Autodesk Fusion 360 part; units mm, degrees
box "BoxPrimitive1" add length 20 width 33 height 3 placed x (0, 0, 1) y (1, 0, 0) z (0, 1, 0) at (0, 0, 0)
sketch "Sketch2" plane through (0, 0, 0) normal (0, -1, 0) x (1, 0, 0)
  line L0 (33, 20) -> (0, 20)
  line L1 (0, 20) -> (0, 0)
  line L2 (0, 0) -> (33, 0)
  line L3 (33, 0) -> (33, 20)
  line L4 (16.5, 20) -> (16.5, 0)
  line L5 (16.5, 0) -> (16.5, 1)
  line L6 (16.5, 1) -> (27, 1)
  line L7 (27, 1) -> (6, 1)
  line L8 (6, 1) -> (6, 13)
  line L9 (6, 13) -> (27, 13)
  line L10 (27, 13) -> (27, 1)
  dimension "d6" = 1
  dimension "d7" = 10.5
  dimension "d8" = 21
  dimension "d9" = 12
extrude "Extrude1" add sketch "Sketch2" along normal blind 3 contours L4 L6 L7 L9 L10 | L4 L7 L8 L9
sketch "Sketch3" plane through (0, -3, 0) normal (0, -1, 0) x (1, 0, 0)
  line L0 (27, 13) -> (6, 13)
  line L1 (6, 13) -> (6, 1)
  line L2 (6, 1) -> (27, 1)
  line L3 (27, 1) -> (27, 13)
  line L4 (16.5, 13) -> (16.5, 1)
  line L5 (6, 7) -> (27, 7)
cylinder "CylinderPrimitive1" add diameter 9 height 2 placed x (1, 0, 0) y (0, 0, 1) z (0, -1, 0) at (16.5, -3, 7)
cylinder "CylinderPrimitive2" cut diameter 1.37 height -2 placed x (1, 0, 0) y (0, 0, 1) z (0, -1, 0) at (16.5, -5, 7)
Can you work these out from the model? Positions are in its coordinate system, mm. A direction names the side the tool comes from. Give positions to 0.01 mm unless a question says otherwise; leave off trailing zeros. Loops run counter-clockwise (first coordinate to the right, second up) from the corner with the lowest first, then second, coordinate; pieces in that order, holes last. Notation, with made-up numbers: M 82,-30 L 93,-30 A24 cw 93,9 Z; hole C -38,-3.75 d10. An arc over 180 degrees is marked long. One line per question, with ' | ' between items. Start each with the question number.
Q1. If we mould it in two halves opening along X, with no side actions, what happens to faces 1 (the flat face through (0, 1, 10)), 2 (the flat face through (16, -3, 7)), 3 (the flat face through (16, 1, 20)), 4 (the flat face through (27, -1, 7))? For each: +X half, -X half, draft (parallel to the pull), parting line (faces both ways), or undercut.
Q2. For pin 1 Ø1.1 at (x, z) = (16.5, 7) entering from -Y; pin 2 Ø0.9 at (x, y) = (17, -2) entering from -Z; pin 3 Ø1.5 at (x, y) = (21, -1.5) entering from +Z, each with a flat end and sliding along its axis, tell me the tip position at first contact or that it passes through.
Q3. For faces 5 (the cylindrical face through (17.15, -4.01, 7.21)), 6 (the flat face through (6, -1, 7)), 7 (the flat face through (16, -1, 13)), which set-ups out of +Z, -Z, +X, -X, +Y, -Y let a thin tool reach every point of the face, with its end or its side?
Q4. If we section it at A-A (x = 16.5): Please give me the cut outline in (y, z) (3 decimals), plus the area to 3 significant figures.
Q5. If I drill on line 1 (Z direction, x = 16.5, y = -4.4) (3 decimals); line 2 (Y direction, x = 4.5, z = 16.75); line 3 (Y direction, x = 26.5, z = 1.5), over which ranges is the centre line in solid material (lowest first)? Write a range as from..to.
Q6. If we section it at B-B (z = 7): Please give me the cut outline in (x, y) (3 decimals), plus the area to 3 significant figures.
Q7. If we section it at D-D (z = 10.25): Please give me the cut outline in (x, y), plus the area to 3 significant figures.
Q8. If we section it at C-C (y = -4): Please give me the cut outline in (x, z) (3 decimals), plus the area to 3 significant figures.
Computed:
1) face 1: -X half | face 2: undercut | face 3: draft | face 4: +X half
2) pin 1: stops at y = -3 | pin 2: stops at z = 1 | pin 3: stops at z = 13
3) face 5: -Y | face 6: +Z, -Z, -X, -Y | face 7: +Z, +X, -X, -Y
4) outline: M -5,2.5 L -3,2.5 L -3,1 L 0,1 L 0,0 L 3,0 L 3,20 L 0,20 L 0,13 L -3,13 L -3,11.5 L -5,11.5 L -5,7.685 L -3,7.685 L -3,6.315 L -5,6.315 Z | area: 111 mm²
5) line 1: z = 2.5..6.315, 7.685..11.5 | line 2: y = 0..3 | line 3: y = -3..3
6) outline: M 0,0 L 6,0 L 6,-3 L 12,-3 L 12,-5 L 15.815,-5 L 15.815,-3 L 17.185,-3 L 17.185,-5 L 21,-5 L 21,-3 L 27,-3 L 27,0 L 33,0 L 33,3 L 0,3 Z | area: 177 mm²
7) outline: M 0,0 L 6,0 L 6,-3 L 13.39,-3 L 13.39,-5 L 19.61,-5 L 19.61,-3 L 27,-3 L 27,0 L 33,0 L 33,3 L 0,3 Z | area: 174 mm²
8) outline: C 16.5,7 d9; hole C 16.5,7 d1.37 | area: 62.1 mm²
